```python
from build123d import *

# Parameters (mm, degrees)
EXTRUSION1_DEPTH = 50
EXTRUSION2_REACH = 3
ESQUISSE2_R      = 1.5
EXTRUSION3_REACH = 13.207
ESQUISSE3_R      = 1.5


with BuildPart() as part:
    # Esquisse1 → Extrusion1 (new body)
    with BuildSketch(Plane(origin=(0, 0, 0), x_dir=(1, 0, 0), z_dir=(0, 1, 0))):
        Polygon((0, 0), (0, 20.414213562), (1, 20.414213562), (1, 0.414213562), (15.142135624, -13.727922061), (14.435028843, -14.435028843), align=None)
    extrude(amount=EXTRUSION1_DEPTH)

    # Esquisse2 → Extrusion2 (cut, up to next)
    with BuildSketch(Plane(origin=(1, 0, 0), x_dir=(0, 0, -1), z_dir=(1, 0, 0)), mode=Mode.PRIVATE) as extrusion2_sk1:
        with Locations((10.414213562, 6.5)):
            Circle(ESQUISSE2_R)
    extrusion2_tool1 = extrude(extrusion2_sk1.sketch, amount=-EXTRUSION2_REACH, mode=Mode.PRIVATE) & part.part
    add(extrusion2_tool1.solids().sort_by_distance((1, 6.5, -10.414214))[0], mode=Mode.SUBTRACT)
    # Esquisse2 → Extrusion2 (cut, up to next)
    with BuildSketch(Plane(origin=(1, 0, 0), x_dir=(0, 0, -1), z_dir=(1, 0, 0)), mode=Mode.PRIVATE) as extrusion2_sk2:
        with Locations((10.414213562, 43.5)):
            Circle(ESQUISSE2_R)
    extrusion2_tool2 = extrude(extrusion2_sk2.sketch, amount=-EXTRUSION2_REACH, mode=Mode.PRIVATE) & part.part
    add(extrusion2_tool2.solids().sort_by_distance((1, 43.5, -10.414214))[0], mode=Mode.SUBTRACT)

    # Esquisse3 → Extrusion3 (cut, up to next)
    with BuildSketch(Plane(origin=(0.707106781, 0, -0.707106781), x_dir=(-0.707106781, 0, -0.707106781), z_dir=(0.707106781, 0, -0.707106781)), mode=Mode.PRIVATE) as extrusion3_sk1:
        with Locations((-10.414213562, 43.5)):
            Circle(ESQUISSE3_R)
    extrusion3_tool1 = extrude(extrusion3_sk1.sketch, amount=-EXTRUSION3_REACH, mode=Mode.PRIVATE) & part.part
    add(extrusion3_tool1.solids().sort_by_distance((8.071068, 43.5, 6.656854))[0], mode=Mode.SUBTRACT)
    # Esquisse3 → Extrusion3 (cut, up to next)
    with BuildSketch(Plane(origin=(0.707106781, 0, -0.707106781), x_dir=(-0.707106781, 0, -0.707106781), z_dir=(0.707106781, 0, -0.707106781)), mode=Mode.PRIVATE) as extrusion3_sk2:
        with Locations((-10.414213562, 6.5)):
            Circle(ESQUISSE3_R)
    extrusion3_tool2 = extrude(extrusion3_sk2.sketch, amount=-EXTRUSION3_REACH, mode=Mode.PRIVATE) & part.part
    add(extrusion3_tool2.solids().sort_by_distance((8.071068, 6.5, 6.656854))[0], mode=Mode.SUBTRACT)


solid = part.part
```
Source: CAD feature listing. Evaluate the final solid. Frame: model axes, mm. A direction names the side the tool comes from. Give positions to 0.01 mm unless a question says otherwise; leave off trailing zeros. Loops run counter-clockwise (first coordinate to the right, second up) from the corner with the lowest first, then second, coordinate; pieces in that order, holes last. Notation, with made-up numbers: (-37, 78.25) -> (13, 78.25) arc R7 ccw to (13, 85.25) -> close; hole circle Ø10 at (87, -19.75). An arc over 180 degrees is marked (long way). Put each result on its own line as item: value. Start each with the question number.
1) Material intervals for probe 1 along X at (y, z) = (5.5, -17); probe 2 along X at (y, z) = (16, 13.5); probe 3 along Z at (x, y) = (9.5, 25), sorted ascending.
2) Contact query for flat-ended pins moving along their axis: P1, Ø10, axis at y = 18, z = -9, coming from the +X side; P2, Ø6, axis at y = 9.5, z = 2.5, coming from the +X side; P3, Ø1.5, axis at y = 26.5, z = 1.5, coming from the +X side. Output: stop coordinate, or through.
3) Cut plane C-C (z = -2). Return loops of the section in (x, y).
4) Draft query along Y for faces 1 (the face through (2, 50, 1)), 2 (the face through (0, 25, -10)), 3 (the face through (7.952, 5.036, 7.235)), 4 (the face through (2, 0, 1)). Return one class per face: released by +Y, released by -Y, zero draft, split by the parting line, or undercut.
5) Reachability of faces 5 (the face through (7, 25, 7)), 6 (the face through (1, 25, -11)) from +Z, -Z, +X, -X, +Y, -Y: full face, straight path, thin tool, end or side. Return the list, or none.
6) Cut plane D-D (x = 8). State how many separate pieces and enclosed holes the cut face has, then the cut area to 3 significant figures.
7) Cut plane A-A (y = 6.5). Return loops of the section in (x, z), then the cut area to 3 significant figures.
8) Cut plane B-B (y = 33). Return loops of the section in (x, z), then the cut area to 3 significant figures.
Results are:
1. probe 1: x = 0 to 1
1. probe 2: x = 13.5 to 14.91
1. probe 3: z = 8.09 to 9.5
2. P1: stops at x = 1
2. P2: stops at x = 6.91
2. P3: stops at x = 3.66
3. outline: (0, 0) -> (1, 0) -> (1, 50) -> (0, 50) -> close
4. face 1: released by +Y
4. face 2: zero draft
4. face 3: undercut
4. face 4: released by -Y
5. face 5: +Z, -X, +Y, -Y
5. face 6: -Z, +X, +Y, -Y
6. separate pieces: 3
6. enclosed holes: 0
6. area: 62.7 mm2
7. outline: (0, -20.41) -> (1, -20.41) -> (1, -11.91) -> (0, -11.91) -> close; (0, -8.91) -> (1, -8.91) -> (1, -0.41) -> (7.01, 5.6) -> (6.3, 6.3) -> (0, 0) -> close; (8.42, 8.42) -> (9.13, 7.72) -> (15.14, 13.73) -> (14.44, 14.44) -> close
7. area: 34.4 mm2
8. outline: (0, -20.41) -> (1, -20.41) -> (1, -0.41) -> (15.14, 13.73) -> (14.44, 14.44) -> (0, 0) -> close
8. area: 40.4 mm2
